Geometry: final body of the model. Coordinates: model frame, mm. Face numbers are marked on the shaded views. A direction names the side the tool comes from. Give positions to 0.01 mm unless a question says otherwise; leave off trailing zeros. Write each loop counter-clockwise with the first axis right and the second up, starting at its lowest first coordinate (ties: lowest second). Pieces come first, ordered by that corner, then holes.
Q1. Section A-A (y = -7.25). State how many separate pieces and enclosed holes the cut face has, plus the area to 3 significant figures.
Q2. Reachability of the marked faces 1 and 2 from +Z, -Z, +X, -X, +Y, -Y: full face, straight path, thin tool, end or side. Return the list, or none.
Q3. Section D-D (z = -3). Return the cut outline in (x, y), plus the area to 3 significant figures.
Q4. Section B-B (z = -9.5). Return the cut outline in (x, y), plus the area to 3 significant figures.
Q5. Mould query, pull axis Y, two halves, no side actions, for the marked faces 3, 4 and 5. Classes: +Y half, -Y half, draft (parallel to the pull), parting line (faces both ways), or undercut.
Q6. Pin query (flat end, axial travel): pin 1 Ø8 at (x, z) = (-1, -14.5) entering from +Y; pin 2 Ø6 at (y, z) = (-1, -14) entering from +X; pin 3 Ø5 at (x, z) = (6.5, -4.5) entering from -Y. Return the tip coordinate at first contact, or that it passes through.
Q7. Line query: line 1 (X direction, y = 0, z = -2.5); line 2 (Y direction, x = 0, z = -14.75); line 3 (X direction, y = 0, z = -9). Output: solid intervals per line, ascending.
from build123d import *

# Parameters (mm, degrees)
CHAMFER1_SIZE = 0.8


with BuildPart() as part:
    # Sketch2 → Revolve1 (revolve)
    with BuildSketch(Plane(origin=(0, 0, 0), x_dir=(1, 0, 0), z_dir=(0, 1, 0))):
        Polygon((1.65, 18.8), (1.65, 0), (9.5, 0), (9.5, 2), (6, 2), (6, 3.5), (8.5, 3.5), (8.5, 4.4), (3.5, 4.4), (3.5, 5.9), (8.5, 5.9), (8.5, 6.8), (3.5, 6.8), (3.5, 8.3), (8.5, 8.3), (8.5, 9.2), (3.5, 9.2), (3.5, 10.7), (8.5, 10.7), (8.5, 11.6), (3.5, 11.6), (3.5, 13.1), (8.5, 13.1), (8.5, 14), (3.5, 14), (3.5, 15.5), (8.5, 15.5), (8.5, 16.4), (3.5, 16.4), (3.5, 17.9), (8.5, 17.9), (8.5, 18.8), align=None)
    revolve(axis=Axis((0, 0, 0), (0, 0, -1)))

    # Chamfer1
    chamfer1_edges = [part.edges().sort_by_distance(p)[0] for p in [
        (-1.65, 0, 0),
    ]]
    chamfer(chamfer1_edges, length=CHAMFER1_SIZE)


solid = part.part
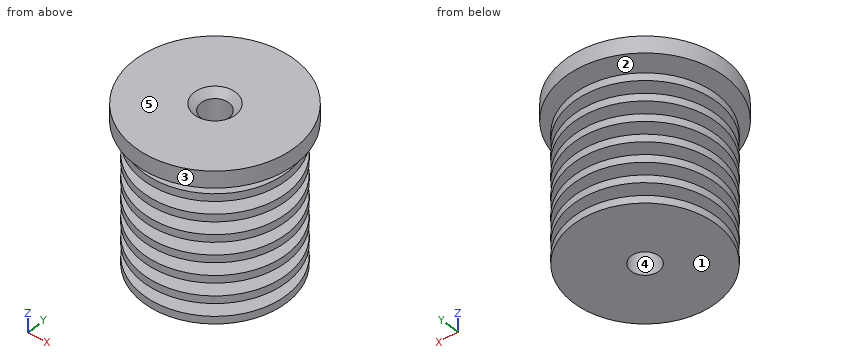
Computed:
1. separate pieces: 8
1. enclosed holes: 0
1. area: 80.5 mm2
2. face 1: -Z, +X, -X, +Y, -Y
2. face 2: none
3. outline: circle Ø12 at (0, 0); hole circle Ø3.3 at (0, 0)
3. area: 105 mm2
4. outline: circle Ø7 at (0, 0); hole circle Ø3.3 at (0, 0)
4. area: 29.9 mm2
5. face 3: parting line
5. face 4: undercut
5. face 5: draft
6. pin 1: stops at y = 8.5
6. pin 2: stops at x = 8.5
6. pin 3: stops at y = -7.5
7. line 1: x = -6 to -1.65, 1.65 to 6
7. line 2: y = -3.5 to -1.65, 1.65 to 3.5
7. line 3: x = -8.5 to -1.65, 1.65 to 8.5
